For this review, take the finished solid that the model builds, in its own axes (mm). Coordinates: 2 decimals unless noted, no trailing zeros. Loops run counter-clockwise (first coordinate to the right, second up) from the corner with the lowest first, then second, coordinate; pieces in that order, holes last. Notation, with made-up numbers: (49.5, -8) - (102.5, -8) arc R21 cw to (102.5, 18) - close; hole circle Ø4 at (85.25, 58). An arc over 180 degrees is marked (long way). Answer as a JSON object with one key per item and string values. Group by question number.
Item 1: We need section C-C (z = 2.55). State how many separate pieces and enclosed holes the cut face has, then the cut area to 3 significant figures.
Item 2: We need section A-A (y = -65.5). Give the boundary of the cut face in (x, z), then the cut area to 3 significant figures.
Item 3: We need section B-B (y = 70.5). Give the boundary of the cut face in (x, z).
Item 4: Clearance check with flat-ended pins moving along their axes: pin 1 (1 mm diameter, centred on y = 33.5, z = 1, fed in from -X); pin 2 (1.6 mm diameter, centred on y = -98, z = 2, fed in from +X); pin 3 (0.9 mm diameter, centred on x = 2.5, z = 1.5, fed in from +Y). State where each tip first meets the part, or that it passes through.
Item 5: To check wall thickness, follow line 1 (X direction, y = -62.5, z = 2.75); line 2 (X direction, y = 89, z = 1.9); line 3 (X direction, y = -25.5, z = 0.3). State the ranges of each line that lie inside material, in increasing order.
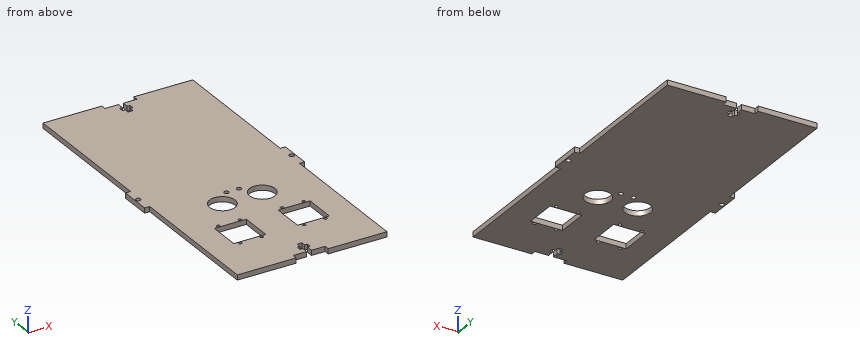
from build123d import *

# Parameters (mm, degrees)
SKETCH1_W           = 100
SKETCH1_H           = 200
BOSS_EXTRUDE2_DEPTH = 3.18
SKETCH2_R           = 1.55
SKETCH2_W           = 3.18
SKETCH2_H           = 90.125
CUT_EXTRUDE1_DEPTH  = 4.18
SKETCH4_R           = 1
CUT_EXTRUDE15_DEPTH = 10
SKETCH5_R           = 8
CUT_EXTRUDE16_DEPTH = 4.18
SKETCH6_R           = 1.47
CUT_EXTRUDE17_DEPTH = 4.18
SKETCH7_W           = 20
SKETCH7_H           = 20
CUT_EXTRUDE18_DEPTH = 4.18


with BuildPart() as part:
    # Sketch1 → Boss-Extrude2 (new body)
    with BuildSketch(Plane.XY):
        Rectangle(SKETCH1_W, SKETCH1_H)
    extrude(amount=BOSS_EXTRUDE2_DEPTH)

    # Sketch2 → Cut-Extrude1 (cut, through all)
    with BuildSketch(Plane.XY.offset(3.18)):
        with Locations((-48, 0)):
            Circle(SKETCH2_R)
        Polygon((-10, 100), (-10, 96.82), (-1.5, 96.82), (-1.5, 92.82), (-3.25, 92.82), (-3.25, 89.82), (-1.5, 89.82), (-1.5, 87), (1.5, 87), (1.5, 89.82), (3.25, 89.82), (3.25, 92.82), (1.5, 92.82), (1.5, 96.82), (10, 96.82), (10, 100), align=None)
        with Locations((-48.41, 54.9375)):
            Rectangle(SKETCH2_W, SKETCH2_H)
        with Locations((-48.41, -54.9375)):
            Rectangle(SKETCH2_W, SKETCH2_H)
    cut_extrude1 = extrude(amount=-CUT_EXTRUDE1_DEPTH, mode=Mode.SUBTRACT)

    # Mirror1: Cut-Extrude1 across plane
    add(cut_extrude1.mirror(Plane.ZX), mode=Mode.SUBTRACT)

    # Mirror3: Cut-Extrude1 across plane
    add(cut_extrude1.mirror(Plane(origin=(0, 0, 0), x_dir=(0, 0, 1), z_dir=(1, 0, 0))), mode=Mode.SUBTRACT)

    # Sketch4 → Cut-Extrude15 (cut)
    with BuildSketch(Plane(origin=(0, 0, 0), x_dir=(-1, 0, 0), z_dir=(0, 0, -1))):
        with Locations((13.361708712, -70.119061845)):
            Circle(SKETCH4_R)
        with Locations((26.861708712, -70.119061845)):
            Circle(SKETCH4_R)
        with Locations((26.861708712, -47.659061845)):
            Circle(SKETCH4_R)
        with Locations((13.361708712, -47.659061845)):
            Circle(SKETCH4_R)
        with Locations((-12.978894748, -47.682446814)):
            Circle(SKETCH4_R)
        with Locations((-26.478894748, -47.682446814)):
            Circle(SKETCH4_R)
        with Locations((-26.478894748, -70.142446814)):
            Circle(SKETCH4_R)
        with Locations((-12.978894748, -70.142446814)):
            Circle(SKETCH4_R)
    extrude(amount=-CUT_EXTRUDE15_DEPTH, mode=Mode.SUBTRACT)

    # Sketch5 → Cut-Extrude16 (cut, through all)
    with BuildSketch(Plane(origin=(0, 0, 0), x_dir=(-1, 0, 0), z_dir=(0, 0, -1))):
        with Locations((12.031607873, -27.34212165)):
            Circle(SKETCH5_R)
        with Locations((-12.968392127, -27.34212165)):
            Circle(SKETCH5_R)
    extrude(amount=-CUT_EXTRUDE16_DEPTH, mode=Mode.SUBTRACT)

    # Sketch6 → Cut-Extrude17 (cut, through all)
    with BuildSketch(Plane(origin=(0, 0, 0), x_dir=(-1, 0, 0), z_dir=(0, 0, -1))):
        with Locations((3.495113066, -17.537619805)):
            Circle(SKETCH6_R)
        with Locations((-4.43189732, -17.537619805)):
            Circle(SKETCH6_R)
    extrude(amount=-CUT_EXTRUDE17_DEPTH, mode=Mode.SUBTRACT)

    # Sketch7 → Cut-Extrude18 (cut, through all)
    with BuildSketch(Plane(origin=(0, 0, 0), x_dir=(-1, 0, 0), z_dir=(0, 0, -1))):
        with Locations((20.111708712, -58.889061845)):
            Rectangle(SKETCH7_W, SKETCH7_H)
        with Locations((-19.728894748, -58.912446814)):
            Rectangle(SKETCH7_W, SKETCH7_H)
    extrude(amount=-CUT_EXTRUDE18_DEPTH, mode=Mode.SUBTRACT)


solid = part.part
Check sheet entries:
{
 "1": {"separate pieces": "1", "enclosed holes": "16", "area": "17,400 mm2"},
 "2": {"outline": "(-46.82, 0) - (-30.11, 0) - (-30.11, 3.18) - (-46.82, 3.18) - close; (-10.11, 0) - (9.73, 0) - (9.73, 3.18) - (-10.11, 3.18) - close; (29.73, 0) - (46.82, 0) - (46.82, 3.18) - (29.73, 3.18) - close", "area": "171 mm2"},
 "3": {"outline": "(-46.82, 0) - (46.82, 0) - (46.82, 3.18) - (-46.82, 3.18) - close"},
 "4": {"pin 1": "stops at x = -46.82", "pin 2": "stops at x = 46.82", "pin 3": "stops at y = 96.82"},
 "5": {"line 1": "x = -46.82 to -30.11, -10.11 to 9.73, 29.73 to 46.82", "line 2": "x = -46.82 to -1.5, 1.5 to 46.82", "line 3": "x = -46.82 to -19.82, -4.25 to 5.18, 20.75 to 46.82"}
}
